```python
from build123d import *

# Parameters (mm, degrees)
F0_W     = 15.24
F0_H     = 6.35
F1_DEPTH = 177.8
F2_R     = 2.38125
F3_DEPTH = 15.241
F4_R     = 15.875
F5_DEPTH = 10.16
F6_R     = 13.97
F7_DEPTH = 8.89


with BuildPart() as f1:
    # F0 (on Front) → F1 (new body)
    with BuildSketch(Plane.XZ):
        with Locations((1.199444, 3.175)):
            Rectangle(F0_W, F0_H)
    extrude(amount=F1_DEPTH)

    # F2 (on face) → F3 (cut, through all)
    with BuildSketch(Plane.YZ.offset(8.819444)):
        with Locations((-120.65, 3.175)):
            Circle(F2_R)
    extrude(amount=-F3_DEPTH, mode=Mode.SUBTRACT)

    # F4 (on face) → F5 (join)
    with BuildSketch(Plane.XY.offset(6.35)):
        with Locations((1.199444, -12.7)):
            Circle(F4_R)
    extrude(amount=F5_DEPTH)

    # F6 (on face) → F7 (cut)
    with BuildSketch(Plane.XY.offset(16.51)):
        with Locations((1.199444, -12.7)):
            Circle(F6_R)
    extrude(amount=-F7_DEPTH, mode=Mode.SUBTRACT)


solid = f1.part
```
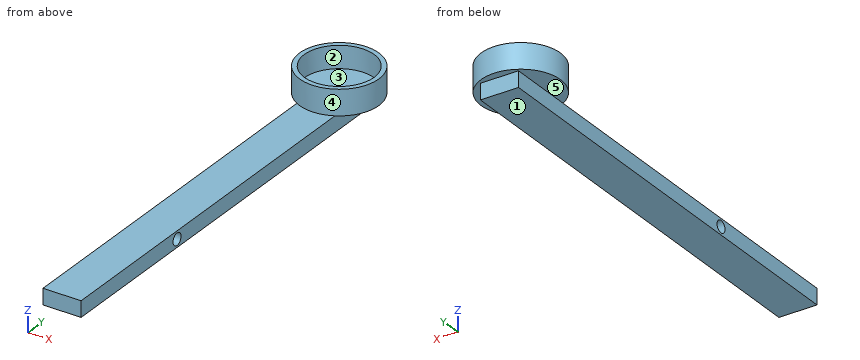
Source: CAD feature listing. Evaluate the final solid. Frame: model axes, mm. Face numbers are marked on the shaded views. A direction names the side the tool comes from. Give positions to 0.01 mm unless a question says otherwise; leave off trailing zeros. Write each loop counter-clockwise with the first axis right and the second up, starting at its lowest first coordinate (ties: lowest second). Pieces come first, ordered by that corner, then holes. Notation, with made-up numbers: (56, 41) - (83, 41) arc R23 cw to (83, 52) - close; hole circle Ø9 at (9, 83). An arc over 180 degrees is marked (long way). One line per item, written item: value. Start each with the question number.
Q1. Section query B-B, the plane y = -12.7. Return the cut outline in (x, z), then the cut area to 3 significant figures.
Q2. Set-up query: the marked faces 1 and 2. Return all of +Z, -Z, +X, -X, +Y, -Y with unobstructed straight access to the full face (end or side cutting, diameter ignored); none if empty.
Q3. Section query A-A, the plane y = -120.65. Return the cut outline in (x, z), then the cut area to 3 significant figures.
Q4. First-contact query: pin 1 Ø12 at (x, y) = (1, -129.5) entering from +Z; pin 2 Ø8.5 at (x, y) = (-4, -12.5) entering from +Z; pin 3 Ø1 at (x, z) = (-8.5, 10.5) entering from -Y; pin 4 Ø4 at (y, z) = (-120.65, 3.175) entering from +X. Flat tips, straight axial feed; report the tip coordinate or a pass-through.
Q5. Draft query along X for the marked faces 3, 4 and 5. Return one class per face: +X half, -X half, draft (parallel to the pull), parting line (faces both ways), or undercut.
Q6. Section query D-D, the plane z = 10. Return the cut outline in (x, y) (3 decimals).
Q7. Material intervals for probe 1 along Z at (x, y) = (-0.75, -120.65); probe 2 along Z at (x, y) = (-6, -131); probe 3 along X at (y, z) = (-21, 16), sorted ascending. Write a range as from..to.
Answer:
1. outline: (-14.68, 6.35) - (-6.42, 6.35) - (-6.42, 0) - (8.82, 0) - (8.82, 6.35) - (17.07, 6.35) - (17.07, 16.51) - (15.17, 16.51) - (15.17, 7.62) - (-12.77, 7.62) - (-12.77, 16.51) - (-14.68, 16.51) - close
1. area: 171 mm2
2. face 1: -Z, +X, -X, +Y, -Y
2. face 2: +Z
3. outline: (-6.42, 0) - (8.82, 0) - (8.82, 0.79) - (-6.42, 0.79) - close; (-6.42, 5.56) - (8.82, 5.56) - (8.82, 6.35) - (-6.42, 6.35) - close
3. area: 24.2 mm2
4. pin 1: stops at z = 6.35
4. pin 2: stops at z = 7.62
4. pin 3: stops at y = -25.64
4. pin 4: passes through
5. face 3: undercut
5. face 4: parting line
5. face 5: draft
6. outline: circle Ø31.75 at (1.199, -12.7); hole circle Ø27.94 at (1.199, -12.7)
7. probe 1: z = 0..0.79, 5.56..6.35
7. probe 2: z = 0..6.35
7. probe 3: x = -12.33..-10.04, 12.44..14.73
